Geometry check sheet. Reference: the model listing, model coordinates, mm. A direction names the side the tool comes from. Coordinates: 2 decimals unless noted, no trailing zeros. Loops run counter-clockwise (first coordinate to the right, second up) from the corner with the lowest first, then second, coordinate; pieces in that order, holes last.
from build123d import *

# Parameters (mm, degrees)
F0_W     = 30
F0_H     = 34
F1_DEPTH = 12
F2_R     = 2.25
F3_DEPTH = 12.001
F4_R     = 4
F5_DEPTH = 12.5
F6_R     = 1.5
F7_DEPTH = 6


with BuildPart() as f1:
    # F0 (on Top) → F1 (new body)
    with BuildSketch(Plane.XY):
        with Locations((15, 17)):
            Rectangle(F0_W, F0_H)
    extrude(amount=F1_DEPTH)

    # F2 (on face) → F3 (cut, through all)
    with BuildSketch(Plane.XY.offset(12)):
        with Locations((6, 29)):
            Circle(F2_R)
        with Locations((24, 29)):
            Circle(F2_R)
        with Locations((24, 5)):
            Circle(F2_R)
        with Locations((6, 5)):
            Circle(F2_R)
    extrude(amount=-F3_DEPTH, mode=Mode.SUBTRACT)

    # F4 (on face) → F5 (cut)
    with BuildSketch(Plane.XZ):
        with Locations((15, 6)):
            Circle(F4_R)
    extrude(amount=-F5_DEPTH, mode=Mode.SUBTRACT)

    # F6 (on face) → F7 (cut)
    with BuildSketch(Plane.XY.offset(12)):
        with Locations((15, 4)):
            Circle(F6_R)
    extrude(amount=-F7_DEPTH, mode=Mode.SUBTRACT)


solid = f1.part
(1) Draft check along Y on faces 4 (the cylindrical face through (8.146, 5.676, 6.084)), 5 (the flat face through (15, 12.5, 6)), 6 (the flat face through (15, 34, 6)). Enter one of: +Y half, -Y half, draft (parallel to the pull), parting line (faces both ways), or undercut.
Findings:
face 4: undercut
face 5: -Y half
face 6: +Y half
(2) Sectioned sample at A-A on z = 6. Record the cut outline in (x, y), and give its area (3 significant figures).
Findings:
outline: (0, 0) - (11, 0) - (11, 12.5) - (19, 12.5) - (19, 0) - (30, 0) - (30, 34) - (0, 34) - close; hole circle Ø4.5 at (6, 5); hole circle Ø4.5 at (6, 29); hole circle Ø4.5 at (24, 5); hole circle Ø4.5 at (24, 29)
area: 856 mm2
(3) Gauge pin test, flat end, axial feed: pin 1 Ø2.5 at (x, z) = (15.5, 6) entering from -Y. Record the tip position at first contact, or that the pin passes through.
Findings:
pin 1: stops at y = 12.5
(4) Sectioned sample at D-D on x = 15. Record the cut outline in (y, z).
Findings:
outline: (0, 0) - (34, 0) - (34, 12) - (5.5, 12) - (5.5, 10) - (12.5, 10) - (12.5, 2) - (0, 2) - close; (0, 10) - (2.5, 10) - (2.5, 12) - (0, 12) - close
(5) Scan lines: L1, parallel to Y at x = 6, z = 2.5; L2, parallel to Y at x = 15, z = 10.8; L3, parallel to X at y = 10, z = 6.25. Record each from-to range of solid material in increasing order.
Findings:
L1: y = 0 to 2.75, 7.25 to 26.75, 31.25 to 34
L2: y = 0 to 2.5, 5.5 to 34
L3: x = 0 to 11.01, 18.99 to 30
(6) Access from +Z, -Z, +X, -X, +Y, -Y to the whole of each face (thin tool, end or side, straight path). Record for faces 1 (the flat face through (30, 17, 6)), 2 (the cylindrical face through (13.5, 4.07, 10.87)), 3 (the cylindrical face through (14.133, 6.162, 2.095)).
Findings:
face 1: +Z, -Z, +X, +Y, -Y
face 2: +Z
face 3: -Y
(7) Sectioned sample at C-C on y = 4. Record the cut outline in (x, z).
Findings:
outline: (0, 0) - (3.98, 0) - (3.98, 12) - (0, 12) - close; (8.02, 0) - (21.98, 0) - (21.98, 12) - (16.5, 12) - (16.5, 9.71) arc R4 cw (long way) to (13.5, 9.71) - (13.5, 12) - (8.02, 12) - close; (26.02, 0) - (30, 0) - (30, 12) - (26.02, 12) - close
(8) Sectioned sample at B-B on x = 6. Record the cut outline in (y, z).
Findings:
outline: (0, 0) - (2.75, 0) - (2.75, 12) - (0, 12) - close; (7.25, 0) - (26.75, 0) - (26.75, 12) - (7.25, 12) - close; (31.25, 0) - (34, 0) - (34, 12) - (31.25, 12) - close
